from build123d import *

# Parameters (mm, degrees)
SKETCH1_R           = 3.374999999
SKETCH1_R_2         = 3.375000001
SKETCH1_R_3         = 3.375000002
SKETCH1_R_4         = 3.606945722
SKETCH1_R_5         = 3.951125178
BOSS_EXTRUDE1_DEPTH = 3


with BuildPart() as part:
    # Sketch1 → Boss-Extrude1 (new body)
    with BuildSketch(Plane(origin=(0, 0, 0), x_dir=(1, 0, 0), z_dir=(0, 1, 0))):
        Polygon((-41.199524293, -99.465227688), (-99.465227688, -41.199524293), (-99.465250609, 41.199501372), (-41.199524293, 99.465227688), (99.465250609, 99.465227688), (99.465250609, -99.465227688), align=None)
        with Locations((80.004750061, 86.09025128)):
            Circle(SKETCH1_R, mode=Mode.SUBTRACT)
        with Locations((-6.085500548, 6.7e-07)):
            Circle(SKETCH1_R_2, mode=Mode.SUBTRACT)
        with Locations((80.004750061, -86.090249939)):
            Circle(SKETCH1_R_3, mode=Mode.SUBTRACT)
        with Locations((-79.537020487, -32.945312596)):
            Circle(SKETCH1_R_4, mode=Mode.SUBTRACT)
        with Locations((-60.875, -60.875)):
            Circle(SKETCH1_R_4, mode=Mode.SUBTRACT)
        with Locations((-32.945312596, -79.537020487)):
            Circle(SKETCH1_R_4, mode=Mode.SUBTRACT)
        with Locations((32.945312596, -79.537020487)):
            Circle(SKETCH1_R_4, mode=Mode.SUBTRACT)
        with Locations((60.875, -60.875)):
            Circle(SKETCH1_R_4, mode=Mode.SUBTRACT)
        with Locations((79.537020487, -32.945312596)):
            Circle(SKETCH1_R_4, mode=Mode.SUBTRACT)
        with Locations((86.090250609, 0)):
            Circle(SKETCH1_R_4, mode=Mode.SUBTRACT)
        with Locations((79.537020487, 32.945312596)):
            Circle(SKETCH1_R_4, mode=Mode.SUBTRACT)
        with Locations((60.875, 60.875)):
            Circle(SKETCH1_R_4, mode=Mode.SUBTRACT)
        with Locations((32.945312596, 79.537020487)):
            Circle(SKETCH1_R_4, mode=Mode.SUBTRACT)
        with Locations((0, 86.090250609)):
            Circle(SKETCH1_R_4, mode=Mode.SUBTRACT)
        with Locations((-32.945312596, 79.537020487)):
            Circle(SKETCH1_R_4, mode=Mode.SUBTRACT)
        with Locations((-60.875, 60.875)):
            Circle(SKETCH1_R_4, mode=Mode.SUBTRACT)
        with Locations((-79.537020487, 32.945312596)):
            Circle(SKETCH1_R_4, mode=Mode.SUBTRACT)
        with Locations((-86.090250609, 0)):
            Circle(SKETCH1_R_4, mode=Mode.SUBTRACT)
        with Locations((0, -86.090250609)):
            Circle(SKETCH1_R_5, mode=Mode.SUBTRACT)
    extrude(amount=BOSS_EXTRUDE1_DEPTH)


solid = part.part
Read the model definition and answer for the solid it produces. Units are mm, in the model's axes. Round coordinates to 2 decimals unless told otherwise and drop trailing zeros. Order: outer loops, then holes, each group sorted by start corner. A loop starts at its lowest first (then second) coordinate and runs counter-clockwise, first axis right, second up. Notation, with made-up numbers: (28.25, 86) - (52.25, 86) arc R16 ccw to (52.25, 106) - close; hole circle Ø3 at (-15, 33.25). An arc over 180 degrees is marked (long way). Use one line per item in the form item = value. Start each with the question number.
(1) The part is cut by section D-D (z = 0). Give the vertices of the cut face in (x, y).
(2) Find the intervals of material crossed by line 1 along Z through (x, y) = (0, 2.45); line 2 along Z through (x, y) = (81, 2.6); line 3 along X through (y, z) = (0.8, -64), in increasing order. Write a range as from..to.
(3) The part is cut by section A-A (x = 0). Give the vertices of the cut face in (y, z), then the cut area to 3 significant figures.
(4) Determine the mould class of faces 1 (the face through (82.487, 1.479, -0.159)), 2 (the face through (-69.925, 1.479, 70.74)), 3 (the face through (-0.47, 1.479, -89.667)), 4 (the face through (1, 0, -1)) for opening direction X: +X half, -X half, draft (parallel to the pull), parting line (faces both ways), or undercut.
(5) The part is cut by section C-C (x = -86.5). Give the vertices of the cut face in (y, z).
(6) A flat-ended cylindrical pin translates along its axis: pin 1 Ø8.5 at (x, z) = (0, -86.09) entering from -Y. Find the tip coordinate at first contact, or state that the pin passes through.
(7) The part is cut by section B-B (y = 0.45). Count the separate pieces of the cut face and the enclosed holes in it, then the cut area to 3 significant figures.
Checked values:
q1.outline = (-99.47, 0) - (-89.7, 0) - (-89.7, 3) - (-99.47, 3) - close; (-82.48, 0) - (-9.46, 0) - (-9.46, 3) - (-82.48, 3) - close; (-2.71, 0) - (82.48, 0) - (82.48, 3) - (-2.71, 3) - close; (89.7, 0) - (99.47, 0) - (99.47, 3) - (89.7, 3) - close
q2.line_1 = -99.47..-89.7, -82.48..82.14, 90.04..99.47
q2.line_2 = -99.47..-89.32, -82.87..-36.24, -29.65..29.65, 36.24..82.87, 89.32..99.47
q2.line_3 = -76.66..-62.68, -59.07..59.07, 62.68..99.47
q3.outline = (0, -99.47) - (3, -99.47) - (3, -89.7) - (0, -89.7) - close; (0, -82.48) - (3, -82.48) - (3, 82.14) - (0, 82.14) - close; (0, 90.04) - (3, 90.04) - (3, 99.47) - (0, 99.47) - close
q3.area = 551 mm^2
q4.face_1 = undercut
q4.face_2 = -X half
q4.face_3 = undercut
q4.face_4 = draft
q5.outline = (0, -54.16) - (3, -54.16) - (3, -3.58) - (0, -3.58) - close; (0, 3.58) - (3, 3.58) - (3, 54.16) - (0, 54.16) - close
q6.pin_1 = 0
q7.separate_pieces = 1
q7.enclosed_holes = 19
q7.area = 35,400 mm^2
